```python
from build123d import *

# Parameters (mm, degrees)
SKETCH_W   = 90
SKETCH_H   = 60
SKETCH_R   = 2.25
SKETCH_R_2 = 2
SKETCH_R_3 = 1.5
SKETCH_W_2 = 7
SKETCH_H_2 = 4
SKETCH_W_3 = 19
SKETCH_H_3 = 18
SKETCH_W_4 = 21.8
SKETCH_H_4 = 8
PAD_DEPTH  = 3


with BuildPart() as part:
    # Sketch → Pad (new body)
    with BuildSketch(Plane.XY):
        with Locations((45, 30)):
            Rectangle(SKETCH_W, SKETCH_H)
        with Locations((10, 5)):
            Circle(SKETCH_R, mode=Mode.SUBTRACT)
        with Locations((33, 24)):
            Circle(SKETCH_R_2, mode=Mode.SUBTRACT)
        with Locations((33, 36)):
            Circle(SKETCH_R_2, mode=Mode.SUBTRACT)
        with Locations((33, 30)):
            Circle(SKETCH_R_2, mode=Mode.SUBTRACT)
        with Locations((10, 55)):
            Circle(SKETCH_R, mode=Mode.SUBTRACT)
        with Locations((14, 11)):
            Circle(SKETCH_R_3, mode=Mode.SUBTRACT)
        with Locations((5, 11)):
            Circle(SKETCH_R_3, mode=Mode.SUBTRACT)
        with Locations((14, 49)):
            Circle(SKETCH_R_3, mode=Mode.SUBTRACT)
        with Locations((5, 49)):
            Circle(SKETCH_R_3, mode=Mode.SUBTRACT)
        with Locations((80, 45)):
            Circle(SKETCH_R_3, mode=Mode.SUBTRACT)
        with Locations((29, 4.5)):
            Circle(SKETCH_R_3, mode=Mode.SUBTRACT)
        with Locations((42.8, 4.5)):
            Circle(SKETCH_R_3, mode=Mode.SUBTRACT)
        with Locations((10, 16)):
            Rectangle(SKETCH_W_2, SKETCH_H_2, mode=Mode.SUBTRACT)
        with Locations((10, 44)):
            Rectangle(SKETCH_W_2, SKETCH_H_2, mode=Mode.SUBTRACT)
        with Locations((10.5, 30)):
            Rectangle(SKETCH_W_3, SKETCH_H_3, mode=Mode.SUBTRACT)
        with Locations((35.9, 14.5)):
            Rectangle(SKETCH_W_4, SKETCH_H_4, mode=Mode.SUBTRACT)
    pad = extrude(amount=PAD_DEPTH)

    # Mirrored: Pad across face of Pad
    add(pad.mirror(Plane(origin=(90, 30, 1.5), x_dir=(0, 1, 0), z_dir=(1, 0, 0))))


solid = part.part
```
Can you work these out from the model? Positions are in its coordinate system, mm. A direction names the side the tool comes from. Coordinates: 2 decimals unless noted, no trailing zeros. Order: outer loops, then holes, each group sorted by start corner. A loop starts at its lowest first (then second) coordinate and runs counter-clockwise, first axis right, second up.
1. For faces 4 (the face through (6.5, 44, 1)), 5 (the face through (91, 0, 1)), which set-ups out of +Z, -Z, +X, -X, +Y, -Y let a thin tool reach every point of the face, with its end or its side?
2. If we section it at D-D (x = 10): Please give me the cut outline in (y, z), then the cut area to 3 significant figures.
3. If we section it at A-A (y = 55): Please give me the cut outline in (x, z).
4. I need wall thicknesses on line 1 (Y direction, x = 147, z = 1); line 2 (X direction, y = 14.5, z = 1.6); line 3 (Y direction, x = 14, z = 0.9). Which ranges of each line are inside material? Lowest first, please.
5. If we section it at B-B (x = 33): Please give me the cut outline in (y, z).
6. Thinking about a two-plate mould opening in X: for faces 1 (the face through (180, 30, 1)), 2 (the face through (173.614, 10.425, 1.479)), 3 (the face through (91, 60, 1)), which applies, +X half, -X half, draft (parallel to the pull), parting line (faces both ways), or undercut?
7. If we section it at C-C (y = 36): Please give me the cut outline in (x, z).
8. I'm going to push a flat-ended pin straight in: pin 1 (0.9 mm diameter, centred on x = 169, z = 2, fed in from -Y). Where does the tip first touch, or does it pass through?
Entries:
1. face 4: +Z, -Z
1. face 5: +Z, -Z, +X, -X, -Y
2. outline: (0, 0) - (2.75, 0) - (2.75, 3) - (0, 3) - close; (7.25, 0) - (14, 0) - (14, 3) - (7.25, 3) - close; (18, 0) - (21, 0) - (21, 3) - (18, 3) - close; (39, 0) - (42, 0) - (42, 3) - (39, 3) - close; (46, 0) - (52.75, 0) - (52.75, 3) - (46, 3) - close; (57.25, 0) - (60, 0) - (60, 3) - (57.25, 3) - close
2. area: 75.0 mm2
3. outline: (0, 0) - (7.75, 0) - (7.75, 3) - (0, 3) - close; (12.25, 0) - (167.75, 0) - (167.75, 3) - (12.25, 3) - close; (172.25, 0) - (180, 0) - (180, 3) - (172.25, 3) - close
4. line 1: y = 0 to 10.5, 18.5 to 22, 26 to 28, 32 to 34, 38 to 60
4. line 2: x = 0 to 6.5, 13.5 to 25, 46.8 to 133.2, 155 to 166.5, 173.5 to 180
4. line 3: y = 0 to 9.5, 12.5 to 21, 39 to 47.5, 50.5 to 60
5. outline: (0, 0) - (10.5, 0) - (10.5, 3) - (0, 3) - close; (18.5, 0) - (22, 0) - (22, 3) - (18.5, 3) - close; (26, 0) - (28, 0) - (28, 3) - (26, 3) - close; (32, 0) - (34, 0) - (34, 3) - (32, 3) - close; (38, 0) - (60, 0) - (60, 3) - (38, 3) - close
6. face 1: +X half
6. face 2: undercut
6. face 3: draft
7. outline: (0, 0) - (1, 0) - (1, 3) - (0, 3) - close; (20, 0) - (31, 0) - (31, 3) - (20, 3) - close; (35, 0) - (145, 0) - (145, 3) - (35, 3) - close; (149, 0) - (160, 0) - (160, 3) - (149, 3) - close; (179, 0) - (180, 0) - (180, 3) - (179, 3) - close
8. pin 1: stops at y = 0
